```python
from build123d import *

# Parameters (mm, degrees)
F0_W     = 82.55
F0_H     = 19.05
F1_DEPTH = 63.5
F2_DEPTH = 25.4
F0_W_2   = 25.4
F3_DEPTH = 25.4
F4_DEPTH = 25.4
F0_H_2   = 4.7498
F5_DEPTH = 25.4


with BuildPart() as f1:
    # F0 (on Front) → F1 (new body, symmetric)
    with BuildSketch(Plane.XZ):
        Rectangle(F0_W, F0_H)
    extrude(amount=F1_DEPTH, both=True)

    # F0 (on Front) → F2 (join, symmetric)
    with BuildSketch(Plane.XZ):
        with BuildLine():
            Line((-41.275, 9.525), (41.275, 9.525))
            Line((41.275, 9.525), (41.275, 27.0002))
            ThreePointArc((41.275, 27.0002), (45.9246798487, 38.2255201513), (57.15, 42.8752))
            Line((57.15, 42.8752), (60.325, 42.8752))
            Line((60.325, 42.8752), (60.325, 61.9252))
            Line((60.325, 61.9252), (57.15, 61.9252))
            add(Edge.make_bspline(
                [(-41.275, 9.525), (-41.5499731898, 46.1455024779), (14.5141012144, 61.9252), (57.15, 61.9252)],
                knots=[0, 0, 0, 0, 111.5045361635, 111.5045361635, 111.5045361635, 111.5045361635], degree=3))
        make_face()
    extrude(amount=F2_DEPTH, both=True)

    # F0 (on Front) → F3 (join, symmetric)
    with BuildSketch(Plane.XZ):
        with Locations((73.025, 52.4002)):
            Rectangle(F0_W_2, F0_H)
    extrude(amount=F3_DEPTH, both=True)

    # F0 (on Front) → F4 (join, symmetric)
    with BuildSketch(Plane.XZ):
        Polygon((85.725, 66.675), (85.725, 61.9252), (85.725, 42.8752), (85.725, 38.1), (111.125, 38.1), (111.125, 66.675), align=None)
    extrude(amount=F4_DEPTH, both=True)

    # F0 (on Front) → F5 (join, symmetric)
    with BuildSketch(Plane.XZ):
        with Locations((73.025, 64.3001)):
            Rectangle(F0_W_2, F0_H_2)
    extrude(amount=F5_DEPTH, both=True)


solid = f1.part
```
Input: part model. Units: mm. Frame: model coordinates. A direction names the side the tool comes from. Give positions to 0.01 mm unless a question says otherwise; leave off trailing zeros. Write each loop counter-clockwise with the first axis right and the second up, starting at its lowest first coordinate (ties: lowest second). Pieces come first, ordered by that corner, then holes. Notation, with made-up numbers: (38.5, 3.5) - (53.5, 3.5) arc R22 ccw to (53.5, 26.5) - close; hole circle Ø6 at (77, 22). An arc over 180 degrees is marked (long way). Write item = value, one per line. Start each with the question number.
1) Cut plane A-A (x = 65). Return loops of the section in (y, z) (3 decimals), and give its area (3 significant figures).
2) Pin query (flat end, axial travel): pin 1 (2.5 mm diameter, centred on y = -11, z = 41, fed in from -X); pin 2 (17 mm diameter, centred on x = -2.5, z = 47.5, fed in from +Y); pin 3 (19 mm diameter, centred on x = 8, y = -50.5, fed in from +Z) (3 decimals); pin 4 (12 mm diameter, centred on y = -37, z = 37.5, fed in from +X). Return the tip coordinate at first contact, or that it passes through.
3) Draft query along X for faces 6 (the face through (71, 0, 42.875)), 7 (the face through (41.275, -1, 4)), 8 (the face through (-1, -45, 9.525)), 9 (the face through (85.725, 0, 41)). Return one class per face: pulls with the +X half, pulls with the -X half, needs draft (parallel to the pull), parting line crosses it, or undercut.
4) Material intervals for L1, parallel to Z at x = -1, y = -39.5 (3 decimals); L2, parallel to Z at x = 79, y = 2 (3 decimals); L3, parallel to Y at x = 48, z = 51, sorted ascending. Write a range as [from, to].
5) Cut plane B-B (z = 5.5). Return loops of the section in (x, y) (3 decimals).
6) Reachability of faces 1 (the face through (98, 0, 38.1)), 2 (the face through (-1, 44, 9.525)), 3 (the face through (45.8, -0.4, 38.1)), 4 (the face through (34, -25.4, 39)), 5 (the face through (60.325, 0, 64)) from +Z, -Z, +X, -X, +Y, -Y: full face, straight path, thin tool, end or side. Return the list, or none.
Answers follow:
q1.outline = (-25.4, 42.875) - (25.4, 42.875) - (25.4, 66.675) - (-25.4, 66.675) - close
q1.area = 1,210 mm^2
q2.pin_1 = -24.89
q2.pin_2 = 25.4
q2.pin_3 = 9.525
q2.pin_4 = through
q3.face_6 = undercut
q3.face_7 = pulls with the +X half
q3.face_8 = needs draft
q3.face_9 = undercut
q4.L1 = [-9.525, 9.525]
q4.L2 = [42.875, 66.675]
q4.L3 = [-25.4, 25.4]
q5.outline = (-41.275, -63.5) - (41.275, -63.5) - (41.275, 63.5) - (-41.275, 63.5) - close
q6.face_1 = -Z, +X, +Y, -Y
q6.face_2 = +Z, +X, -X, +Y
q6.face_3 = -Z, +Y, -Y
q6.face_4 = +Z, +X, -X, -Y
q6.face_5 = +Z, -X, +Y, -Y
